Part model, mm, in its own coordinate system. Face numbers are marked on the shaded views. A direction names the side the tool comes from. Round coordinates to 2 decimals unless told otherwise and drop trailing zeros. Loops run counter-clockwise (first coordinate to the right, second up) from the corner with the lowest first, then second, coordinate; pieces in that order, holes last. Notation, with made-up numbers: (-12.75, 50) - (-7.75, 50) arc R24 cw to (-7.75, 65) - close; hole circle Ø1 at (9.25, 44). An arc over 180 degrees is marked (long way). Put each result on its own line as item: value.
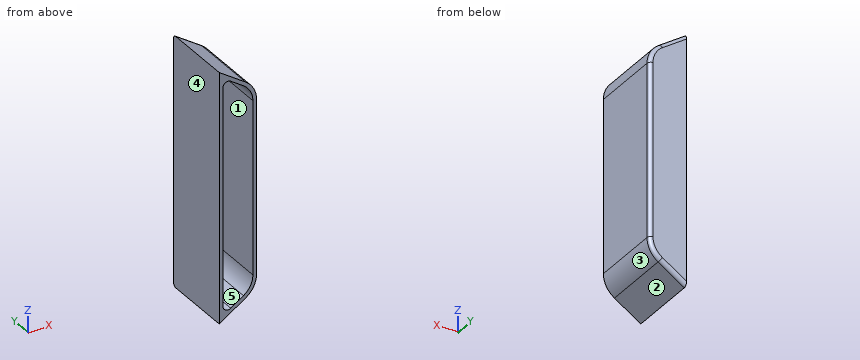
from build123d import *

# Parameters (mm, degrees)
BOSS_EXTRUDE1_DEPTH = 30
SHELL1_T            = -1.5
FILLET1_R           = 2
FILLET2_R           = 1.5


with BuildPart() as part:
    # Sketch1 → Boss-Extrude1 (new body)
    with BuildSketch(Plane(origin=(0, 0, 0), x_dir=(1, 0, 0), z_dir=(0, 1, 0))):
        with BuildLine():
            Line((0, -50), (0, 50))
            Line((0, 50), (10.547001962, 42.968665358))
            ThreePointArc((10.547001962, 42.968665358), (13.816745988, 39.36674167), (15, 34.648162415))
            Line((15, 34.648162415), (15, -34.648162415))
            ThreePointArc((15, -34.648162415), (13.816745988, -39.36674167), (10.547001962, -42.968665358))
            Line((10.547001962, -42.968665358), (0, -50))
        make_face()
    extrude(amount=BOSS_EXTRUDE1_DEPTH)

    # Shell1
    shell1_openings = [part.faces().sort_by_distance(p)[0] for p in [
        (7.177503817, 0, 0),
    ]]
    offset(amount=SHELL1_T, openings=shell1_openings, kind=Kind.INTERSECTION)

    # Fillet1
    fillet1_edges = [part.edges().sort_by_distance(p)[0] for p in [
        (1.5, 14.25, -47.197224362),
        (1.5, 14.25, 47.197224362),
        (5.607475834, 28.5, -44.45890714),
        (1.5, 28.5, 0),
        (5.607475834, 28.5, 44.45890714),
        (12.49423409, 28.5, 38.658954782),
        (13.5, 28.5, 0),
        (12.49423409, 28.5, -38.658954782),
    ]]
    fillet(fillet1_edges, radius=FILLET1_R)

    # Fillet2
    fillet2_edges = [part.edges().sort_by_distance(p)[0] for p in [
        (5.273500981, 30, 46.484332679),
        (13.816745988, 30, 39.36674167),
        (15, 30, 0),
        (13.816745988, 30, -39.36674167),
        (5.273500981, 30, -46.484332679),
    ]]
    fillet(fillet2_edges, radius=FILLET2_R)


solid = part.part
1. Two-plate mould, pull along Z, no slides. Class the marked faces 3, 4 and 5: pulls with the +Z half, pulls with the -Z half, needs draft (parallel to the pull), parting line crosses it, or undercut.
A:
face 3: pulls with the -Z half
face 4: needs draft
face 5: undercut
2. Tool access for the marked faces 1 and 2: list every direction of +Z, -Z, +X, -X, +Y, -Y with a clear straight run to the whole face (end or side of a thin tool).
A:
face 1: -Y
face 2: -Z, +X, +Y, -Y
3. Band-saw the part on B-B (z = -24). List the corners of the cut face in (x, y).
A:
outline: (0, 0) - (1.5, 0) - (1.5, 26.5) arc R2 cw to (3.5, 28.5) - (11.5, 28.5) arc R2 cw to (13.5, 26.5) - (13.5, 0) - (15, 0) - (15, 28.5) arc R1.5 ccw to (13.5, 30) - (0, 30) - close
4. Probe line 1 along X through (y, z) = (20.75, 17); line 2 along Y through (x, z) = (4, -27); line 3 along Y through (x, z) = (13.75, -1). List the from-to ranges inside material, lowest first. Write a range as [from, to].
A:
line 1: x = [0, 1.5], [13.5, 15]
line 2: y = [28.5, 30]
line 3: y = [0, 29.98]
5. Band-saw the part on A-A (y = 10.25). List the corners of the cut face in (x, z).
A:
outline: (0, -50) - (10.55, -42.97) arc R10 ccw to (15, -34.65) - (15, 34.65) arc R10 ccw to (10.55, 42.97) - (0, 50) - close; hole (1.5, -43.46) arc R2 ccw to (4.61, -45.12) - (9.71, -41.72) arc R8.5 ccw to (13.5, -34.65) - (13.5, 34.65) arc R8.5 ccw to (9.71, 41.72) - (4.61, 45.12) arc R2 ccw to (1.5, 43.46) - close
6. Pin check, flat tips, straight feed: P1, Ø4, axis at x = 3.5, y = 12.5, coming from the +Z side; P2, Ø6, axis at x = 10, y = 14.5, coming from the +Z side; P3, Ø3, axis at x = 11.5, z = -23.5, coming from the -Y side. Stop position of each tip, or through.
A:
P1: stops at z = 49
P2: stops at z = 45.33
P3: stops at y = 27.82
